Solid Edge part; units mm, degrees
sketch "Sketch1" plane through (0, 0, 0) normal (0, 0, 1) x (1, 0, 0)
  line L0 (-150, -225) -> (150, -225)
  line L1 (150, -225) -> (150, 225)
  line L2 (150, 225) -> (-150, 225)
  line L3 (-150, 225) -> (-150, -225)
extrude "Protrusion1" add sketch "Sketch1" along normal blind 15
sketch "Sketch2" plane through (0, 0, 15) normal (0, 0, 1) x (1, 0, 0)
  line L0 (-7.5, -285) -> (7.5, -285)
  line L1 (7.5, -285) -> (7.5, -165)
  line L2 (7.5, -165) -> (-7.5, -165)
  line L3 (-7.5, -165) -> (-7.5, -285)
extrude "ExtrudedCutout_1" cut sketch "Sketch2" along normal mid plane 124.4981
sketch "Sketch3" plane through (0, 0, 15) normal (0, 0, 1) x (1, 0, 0)
  circle A0 centre (77.5, -165) radius 5
  circle A1 centre (-77.5, -165) radius 5
  dimension "D1" = 77.5
extrude "ExtrudedCutout_2" cut sketch "Sketch3" along normal mid plane 524.4577
Source: CAD feature listing. Evaluate the final solid. Frame: model axes, mm. A direction names the side the tool comes from. Round coordinates to 2 decimals unless told otherwise and drop trailing zeros. Loops run counter-clockwise (first coordinate to the right, second up) from the corner with the lowest first, then second, coordinate; pieces in that order, holes last.
1. Access query for faces 4 (the flat face through (0, -165, 7)), 5 (the cylindrical face through (82.119, -166.915, 7.605)). Directions: +Z, -Z, +X, -X, +Y, -Y. A direction counts if a zero-diameter tool reaches every point of the face in a straight line with its end or side. Return the directions, or none.
2. Ray query, L1, parallel to Y at x = 77.5, z = 4.75; L2, parallel to Y at x = 73, z = 4.5. Return the intervals inside material, ascending.
3. Mould query, pull axis X, two halves, no side actions, for faces 1 (the flat face through (150, -3, 7)), 2 (the flat face through (7.5, -195, 7)), 3 (the flat face through (-80, -225, 7)). Classes: released by +X, released by -X, zero draft, split by the parting line, or undercut.
4. Section query A-A on x = -77.5. Output: boundary loops of the cut face in (y, z), and give its area (3 significant figures).
5. Contact query for a flat-ended pin moving along its axis: pin 1 (6 mm diameter, centred on x = -77.5, y = -165, fed in from +Z). Output: stop coordinate, or through.
Answers below:
1. face 4: +Z, -Z, -Y
1. face 5: +Z, -Z
2. L1: y = -225 to -170, -160 to 225
2. L2: y = -225 to -167.18, -162.82 to 225
3. face 1: released by +X
3. face 2: undercut
3. face 3: zero draft
4. outline: (-225, 0) - (-170, 0) - (-170, 15) - (-225, 15) - close; (-160, 0) - (225, 0) - (225, 15) - (-160, 15) - close
4. area: 6,600 mm2
5. pin 1: passes through
